Model file for the job. Use its own axes, mm. Face numbers are marked on the shaded views. A direction names the side the tool comes from. Round coordinates to 2 decimals unless told otherwise and drop trailing zeros. Write each loop counter-clockwise with the first axis right and the second up, starting at its lowest first coordinate (ties: lowest second). Pieces come first, ordered by that corner, then holes. Notation, with made-up numbers: (23.25, 37.25) - (49.25, 37.25) arc R20 ccw to (49.25, 51.25) - close; hole circle Ø8 at (45.5, 32). An arc over 180 degrees is marked (long way). Answer as a JSON object with one key per item and string values. Group by question number.
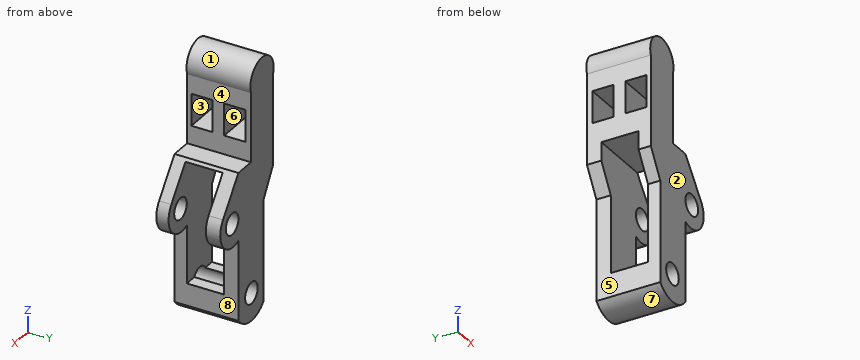
from build123d import *

# Parameters (mm, degrees)
F0_R          = 2
F1_DEPTH      = 12
F2_W          = 4
F2_H          = 6
F3_DEPTH      = 7.197026
F4_W          = 7
F4_H          = 23
F5_DEPTH      = 13.288298
F5_DEPTH_BACK = 25


with BuildPart() as f1:
    # F0 (on Front) → F1 (new body)
    with BuildSketch(Plane.XZ):
        with BuildLine():
            ThreePointArc((3.5, 38.256184), (0, 43.139899), (-3.5, 38.256184))
            Line((-3.5, 38.256184), (-3.5, 21.256184))
            Line((-3.5, 21.256184), (-0.5, 16.256184))
            Line((-0.5, 16.256184), (-0.5, -2.743816))
            ThreePointArc((-0.5, -2.743816), (3.571034, -4.470437), (7.5, -2.44121))
            Line((7.5, -2.44121), (7.5, 12.55879))
            ThreePointArc((7.5, 12.55879), (12.424485, 13.851518), (12.410766, 18.942835))
            Line((12.410766, 18.942835), (7.5, 25.256184))
            Line((7.5, 25.256184), (3.5, 25.256184))
            Line((3.5, 25.256184), (3.5, 38.256184))
        make_face()
        with Locations((3.374378, 0.728549)):
            Circle(F0_R, mode=Mode.SUBTRACT)
        with Locations((9.5, 16.695214)):
            Circle(F0_R, mode=Mode.SUBTRACT)
    extrude(amount=F1_DEPTH)

    # F2 (on face) → F3 (cut, through all)
    with BuildSketch(Plane.YZ.offset(3.5)):
        with Locations((-9.2, 31.756184)):
            Rectangle(F2_W, F2_H)
        with Locations((-3.030456, 31.756184)):
            Rectangle(F2_W, F2_H)
    extrude(amount=-F3_DEPTH, mode=Mode.SUBTRACT)

    # F4 (on Right) → F5 (cut, two sides)
    with BuildSketch(Plane.YZ) as f5_sk:
        with Locations((-6.200001, 13.2)):
            Rectangle(F4_W, F4_H)
    extrude(amount=F5_DEPTH, mode=Mode.SUBTRACT)
    extrude(f5_sk.sketch, amount=-F5_DEPTH_BACK, mode=Mode.SUBTRACT)


solid = f1.part
(1) 3-axis set-ups, long thin cutter, end or side, ignore diameter. For the marked faces 1, 2, 3, 4 and 5: which of +Z, -Z, +X, -X, +Y, -Y reach the whole face in a straight line?
(2) Pull direction Z, two halves, no side cores. Call the marked faces 6, 7 and 8: pulls with the +Z half, pulls with the -Z half, needs draft (parallel to the pull), parting line crosses it, or undercut.
(3) Slice it at C-C (x = 4.5). Write the cut outline in (y, z).
(4) Slice it at D-D (x = 0). Write the cut outline in (y, z), then the cut area to 3 significant figures.
(5) Slice it at A-A (y = -8.25). Write the cut outline in (x, z), then the cut area to 3 significant figures.
(6) Slice it at B-B (z = 11). Write the cut outline in (x, y).
(7) Flat gauge pins, fed straight in: pin 1 (3.5 mm diameter, centred on x = 0, y = -5.5, fed in from -Z); pin 2 (3.5 mm diameter, centred on y = -5.5, z = 31, fed in from +X); pin 3 (1 mm diameter, centred on y = -3, z = 15, fed in from -X); pin 4 (3.5 mm diameter, centred on x = 9.5, z = 16.7, fed in from +Y). Where does each tip first touch, or does it go through?
(8) Drill centre lines: line 1 (Y direction, x = 0.25, z = 29); line 2 (Y direction, x = -0.25, z = 18.5); line 3 (Z direction, x = 1.75, y = -10.75). Where is each one in solid material? Low to high. Write a range as from..to.
Answer:
{
 "1": {"face 1": "+Y, -Y", "face 2": "+Z, -Z, +X, -X, -Y", "face 3": "+X, -X", "face 4": "+X, +Y, -Y", "face 5": "-Z, -X, +Y, -Y"},
 "2": {"face 6": "undercut", "face 7": "pulls with the -Z half", "face 8": "needs draft"},
 "3": {"outline": "(-12, -4.35) - (0, -4.35) - (0, -0.92) - (-12, -0.92) - close; (-12, 2.38) - (-9.7, 2.38) - (-9.7, 24.7) - (-2.7, 24.7) - (-2.7, 2.38) - (0, 2.38) - (0, 25.26) - (-12, 25.26) - close"},
 "4": {"outline": "(-12, -3.23) - (0, -3.23) - (0, 43.14) - (-12, 43.14) - close; hole (-11.2, 28.76) - (-7.2, 28.76) - (-7.2, 34.76) - (-11.2, 34.76) - close; hole (-9.7, 1.7) - (-2.7, 1.7) - (-2.7, 24.7) - (-9.7, 24.7) - close; hole (-5.03, 28.76) - (-1.03, 28.76) - (-1.03, 34.76) - (-5.03, 34.76) - close", "area": "347 mm²"},
 "5": {"outline": "(-3.5, 24.7) - (7.93, 24.7) - (7.5, 25.26) - (3.5, 25.26) - (3.5, 28.76) - (-3.5, 28.76) - close; (-3.5, 34.76) - (3.5, 34.76) - (3.5, 38.26) arc R3.7 ccw (long way) to (-3.5, 38.26) - close; (-0.5, -2.74) arc R5.2 ccw to (7.5, -2.44) - (7.5, 1.7) - (5.12, 1.7) arc R2 cw (long way) to (1.63, 1.7) - (-0.5, 1.7) - close", "area": "120 mm²"},
 "6": {"outline": "(-0.5, -12) - (7.5, -12) - (7.5, -9.7) - (-0.5, -9.7) - close; (-0.5, -2.7) - (7.5, -2.7) - (7.5, 0) - (-0.5, 0) - close"},
 "7": {"pin 1": "z = -4.21", "pin 2": "x = 3.5", "pin 3": "x = -0.5", "pin 4": "through"},
 "8": {"line 1": "-12..-11.2, -7.2..-5.03, -1.03..0", "line 2": "-12..-9.7, -2.7..0", "line 3": "-4.21..-0.44, 1.9..28.76, 34.76..42.7"}
}
